Read the model definition and answer for the solid it produces. Units are mm, in the model's axes. Face numbers are marked on the shaded views. A direction names the side the tool comes from. Coordinates: 2 decimals unless noted, no trailing zeros. Order: outer loops, then holes, each group sorted by start corner. A loop starts at its lowest first (then second) coordinate and runs counter-clockwise, first axis right, second up. Notation, with made-up numbers: M 29,-23 L 75,-23 A30 ccw 75,6 Z; hole C 85.25,36.5 d1. An arc over 180 degrees is marked long. Put each result on its own line as item: value.
from build123d import *

# Parameters (mm, degrees)
SKETCH_5_W                  = 239
SKETCH_5_H                  = 105
EXTRUDE_1_DEPTH             = 20
EXTRUDE_2_DEPTH             = 10
SKETCH_8_W                  = 169
SKETCH_8_H                  = 6
CUT_EXTRUDE_6_DEPTH         = 208.879772946
CUT_EXTRUDE_7_DEPTH         = 204.99509798
CUT_EXTRUDE_7_DEPTH_BACK    = 204.99509798
HOLE_WIZARD_M82_D           = 6.8
HOLE_WIZARD_M82_DEPTH       = 25
HOLE_WIZARD_M82_CSINK_D     = 10
HOLE_WIZARD_M82_CSINK_ANGLE = 90
HOLE_WIZARD_M82_TIP         = 2.042926105
CHAMFER_1_SIZE              = 65
CHAMFER_2_SIZE              = 20
CUT_EXTRUDE_8_DEPTH         = 5
HOLE_WIZARD_M81_D           = 6.8
HOLE_WIZARD_M81_DEPTH       = 23.957073895
HOLE_WIZARD_M81_CSINK_D     = 10
HOLE_WIZARD_M81_CSINK_ANGLE = 90
HOLE_WIZARD_M81_TIP         = 2.042926105
HOLE_WIZARD_M61_D           = 5
HOLE_WIZARD_M61_CSINK_D     = 7
HOLE_WIZARD_M61_CSINK_ANGLE = 90
CUT_EXTRUDE_9_REACH         = 209.88
SKETCH_21_R                 = 20
FILLET_1_R                  = 10
CHAMFER_3_SIZE              = 50
FILLET_2_R                  = 50


with BuildPart() as part:
    # Эскиз5 → Бобышка-Вытянуть1 (new, symmetric)
    with BuildSketch(Plane.XY):
        with Locations((63.5, -32.5)):
            Rectangle(SKETCH_5_W, SKETCH_5_H)
    extrude(amount=EXTRUDE_1_DEPTH, both=True)

    # Эскиз10 → Бобышка-Вытянуть2 (add)
    with BuildSketch(Plane.XY.offset(20)):
        Polygon((-56, 20), (74, 20), (74, -79), (14, -79), (14, -85), (-56, -85), align=None)
    extrude_2 = extrude(amount=EXTRUDE_2_DEPTH)

    # Зеркальное отражение1: Бобышка-Вытянуть2 across plane
    add(extrude_2.mirror(Plane.XY))

    # Эскиз8 → Вырез-Вытянуть6 (cut, through all)
    with BuildSketch(Plane.XY.offset(20)):
        with Locations((98.5, -82)):
            Rectangle(SKETCH_8_W, SKETCH_8_H)
    extrude(amount=-CUT_EXTRUDE_6_DEPTH, mode=Mode.SUBTRACT)

    # Эскиз4 → Вырез-Вытянуть7 (cut, two sides: drawn at the far end of the back side and taken through both)
    with BuildSketch(Plane.XY.offset(-CUT_EXTRUDE_7_DEPTH_BACK)):
        with BuildLine():
            Line((-17.5, 20), (17.5, 20))
            Line((17.5, 20), (17.5, -17.853571071))
            ThreePointArc((17.5, -17.853571071), (0, -25), (-17.5, -17.853571071))
            Line((-17.5, -17.853571071), (-17.5, 20))
        make_face()
    extrude(amount=CUT_EXTRUDE_7_DEPTH + CUT_EXTRUDE_7_DEPTH_BACK, mode=Mode.SUBTRACT)

    # Отверстие обработанное метчиком M82
    with Locations(Plane(origin=(0, -79, 0), x_dir=(-1, 0, 0), z_dir=(0, -1, 0))):
        with Locations((-29, 17.5), (-29, -17.5), (-79, 0), (-169, 0)):
            CounterSinkHole(HOLE_WIZARD_M82_D / 2, HOLE_WIZARD_M82_CSINK_D / 2, depth=HOLE_WIZARD_M82_DEPTH, counter_sink_angle=HOLE_WIZARD_M82_CSINK_ANGLE)
            with Locations((0, 0, -(HOLE_WIZARD_M82_DEPTH + HOLE_WIZARD_M82_TIP / 2))):  # 118° drill point
                Cone(0, HOLE_WIZARD_M82_D / 2, HOLE_WIZARD_M82_TIP, mode=Mode.SUBTRACT)

    # Фаска1
    chamfer_1_edges = [part.edges().sort_by_distance(p)[0] for p in [
        (183, 20, 0),
    ]]
    chamfer(chamfer_1_edges, length=CHAMFER_1_SIZE)

    # Фаска2
    chamfer_2_edges = [part.edges().sort_by_distance(p)[0] for p in [
        (74, 20, 25),
        (74, 20, -25),
    ]]
    chamfer(chamfer_2_edges, length=CHAMFER_2_SIZE)

    # Эскиз14 → Вырез-Вытянуть8 (cut)
    with BuildSketch(Plane.XY.offset(20)):
        Polygon((118, 20), (103, 20), (103, -10), (148, -10), align=None)
    cut_extrude_8 = extrude(amount=-CUT_EXTRUDE_8_DEPTH, mode=Mode.SUBTRACT)

    # Отверстие обработанное метчиком M81
    with Locations(Plane(origin=(0, 20, 0), x_dir=(1, 0, 0), z_dir=(0, 1, 0))):
        with Locations((-30, -15), (30, -15), (-30, 15), (30, 15)):
            CounterSinkHole(HOLE_WIZARD_M81_D / 2, HOLE_WIZARD_M81_CSINK_D / 2, depth=HOLE_WIZARD_M81_DEPTH, counter_sink_angle=HOLE_WIZARD_M81_CSINK_ANGLE)
            with Locations((0, 0, -(HOLE_WIZARD_M81_DEPTH + HOLE_WIZARD_M81_TIP / 2))):  # 118° drill point
                Cone(0, HOLE_WIZARD_M81_D / 2, HOLE_WIZARD_M81_TIP, mode=Mode.SUBTRACT)

    # Зеркальное отражение2: Вырез-Вытянуть8 across plane
    add(cut_extrude_8.mirror(Plane.XY), mode=Mode.SUBTRACT)

    # Отверстие обработанное метчиком M61 (through all)
    with Locations(Plane.XY.offset(20)):
        with Locations((87, -54), (87, 6)):
            hole_wizard_m61 = CounterSinkHole(HOLE_WIZARD_M61_D / 2, HOLE_WIZARD_M61_CSINK_D / 2, counter_sink_angle=HOLE_WIZARD_M61_CSINK_ANGLE)

    # Зеркальное отражение3: Отверстие обработанное метчиком M61 across plane
    add(hole_wizard_m61.mirror(Plane.XY), mode=Mode.SUBTRACT)

    # Эскиз21 → Вырез-Вытянуть9 (cut, up to next)
    with BuildSketch(Plane.XY.offset(20), mode=Mode.PRIVATE) as cut_extrude_9_sk1:
        with Locations((128, -44)):
            Circle(SKETCH_21_R)
    cut_extrude_9_tool1 = extrude(cut_extrude_9_sk1.sketch, amount=-CUT_EXTRUDE_9_REACH, mode=Mode.PRIVATE) & part.part
    add(cut_extrude_9_tool1.solids().sort_by_distance((128, -44, 20))[0], mode=Mode.SUBTRACT)

    # Скругление1
    fillet_1_edges = [part.edges().sort_by_distance(p)[0] for p in [
        (103, -10, 17.5),
        (103, -10, -17.5),
    ]]
    fillet(fillet_1_edges, radius=FILLET_1_R)

    # Фаска3
    chamfer_3_edges = [part.edges().sort_by_distance(p)[0] for p in [
        (-56, -85, 0),
    ]]
    chamfer(chamfer_3_edges, length=CHAMFER_3_SIZE)

    # Скругление2
    fillet_2_edges = [part.edges().sort_by_distance(p)[0] for p in [
        (-56, -35, 0),
    ]]
    fillet(fillet_2_edges, radius=FILLET_2_R)


solid = part.part
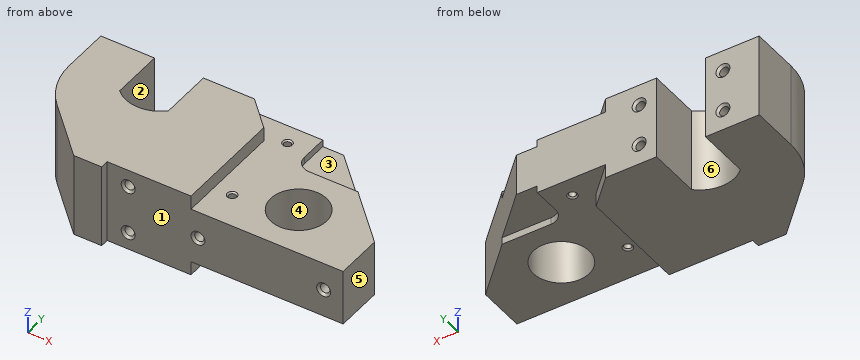
Q1. Consider line 1 along Z through (x, y) = (30, 7); line 2 along X through (y, z) = (8, 13); line 3 along Z through (x, y) = (169, -64.25). Determine where each line is inside the solid, lowest interval first.
Answers below:
line 1: z = -30 to -18.4, -11.6 to 11.6, 18.4 to 30
line 2: x = -56 to -32.75, -27.25 to -17.5, 17.5 to 27.25, 32.75 to 85.5, 88.5 to 130
line 3: z = -20 to -3.4, 3.4 to 20
Q2. A tool of negligible diameter and unlimited length cuts with its end or side. For the marked faces 1, 2 and 3, from which of +Z, -Z, +X, -X, +Y, -Y can it reach the whole face along a straight path? Write none if from no direction.
Answers below:
face 1: +Z, -Z, +X, -Y
face 2: +Z, -Z, +Y
face 3: +Z, +X, +Y
Q3. Find section B-B on y = 6. Write down the section's boundary in (x, z), plus the area to 3 significant figures.
Answers below:
outline: M -56,-30 L -17.5,-30 L -17.5,30 L -56,30 Z; M 17.5,-30 L 68,-30 L 68,-20 L 83.5,-20 L 84.5,-19 L 84.5,19 L 83.5,20 L 68,20 L 68,30 L 17.5,30 Z; M 89.5,-19 L 90.5,-20 L 103,-20 L 103,-15 L 132,-15 L 132,15 L 103,15 L 103,20 L 90.5,20 L 89.5,19 Z; hole C -30,-15 d6.8; hole C -30,15 d6.8; hole C 30,-15 d6.8; hole C 30,15 d6.8
area: 7,260 mm^2
Q4. Find section A-A on x = 87. Write down the section's boundary in (y, z).
Answers below:
outline: M -79,-20 L -57.5,-20 L -56.5,-19 L -56.5,19 L -57.5,20 L -79,20 Z; M -51.5,-19 L -50.5,-20 L 2.5,-20 L 3.5,-19 L 3.5,19 L 2.5,20 L -50.5,20 L -51.5,19 Z; M 8.5,-19 L 9.5,-20 L 20,-20 L 20,20 L 9.5,20 L 8.5,19 Z
Q5. Given pin 1 (4 mm diameter, centred on y = -7, z = -17.5, fed in from +X); pin 2 (8 mm diameter, centred on x = 30, z = 15, fed in from +Y); pin 3 (1 mm diameter, centred on x = 151.5, z = 15.5, fed in from +Y), each flat-ended and moving along its own axis, determine where each tip first touches the part or whether it passes through.
Answers below:
pin 1: stops at x = 108.64
pin 2: stops at y = 19
pin 3: stops at y = -13
Q6. For a pull along Y with two mould halves and no side action, classify the marked faces 4, 5 and 6 as +Y half, -Y half, draft (parallel to the pull), parting line (faces both ways), or undercut.
Answers below:
face 4: undercut
face 5: draft
face 6: +Y half
